Model file for the job. Use its own axes, mm. Face numbers are marked on the shaded views. Coordinates: 2 decimals unless noted, no trailing zeros. Write each loop counter-clockwise with the first axis right and the second up, starting at its lowest first coordinate (ties: lowest second). Pieces come first, ordered by that corner, then holes. Notation, with made-up numbers: (10.5, 80) -> (53.5, 80) arc R16 ccw to (53.5, 94) -> close; hole circle Ø3 at (32.5, -1). An arc over 180 degrees is marked (long way). Answer as a JSON object with one key per item and string values. Group by question number.
from build123d import *

# Parameters (mm, degrees)
SKETCH1_W           = 59.999999888
SKETCH1_H           = 29.999999944
SKETCH1_R           = 6.35889
SKETCH1_R_2         = 2.499999953
BOSS_EXTRUDE1_DEPTH = 6.35
SKETCH2_R           = 9.53389
SKETCH2_R_2         = 6.35889
BOSS_EXTRUDE2_DEPTH = 25.4
FILLET1_R           = 1.27


with BuildPart() as part:
    # Sketch1 → Boss-Extrude1 (new body)
    with BuildSketch(Plane(origin=(0, 0, 0), x_dir=(1, 0, 0), z_dir=(0, 1, 0))):
        Rectangle(SKETCH1_W, SKETCH1_H)
        with Locations(Location((0, 0, 0), (0, 0, 270))):
            Circle(SKETCH1_R, mode=Mode.SUBTRACT)
        with Locations(Location((-25.554999944, 10.554999972, 0), (0, 0, 270))):
            Circle(SKETCH1_R_2, mode=Mode.SUBTRACT)
        with Locations(Location((25.554999944, 10.554999972, 0), (0, 0, 270))):
            Circle(SKETCH1_R_2, mode=Mode.SUBTRACT)
        with Locations(Location((25.554999944, -10.554999972, 0), (0, 0, 270))):
            Circle(SKETCH1_R_2, mode=Mode.SUBTRACT)
        with Locations(Location((-25.554999944, -10.554999972, 0), (0, 0, 270))):
            Circle(SKETCH1_R_2, mode=Mode.SUBTRACT)
    extrude(amount=BOSS_EXTRUDE1_DEPTH)

    # Sketch2 → Boss-Extrude2 (add)
    with BuildSketch(Plane(origin=(0, 6.35, 0), x_dir=(1, 0, 0), z_dir=(0, 1, 0))):
        with Locations(Location((0, 0, 0), (0, 0, 270))):
            Circle(SKETCH2_R)
        with Locations(Location((0, 0, 0), (0, 0, 270))):
            Circle(SKETCH2_R_2, mode=Mode.SUBTRACT)
    extrude(amount=BOSS_EXTRUDE2_DEPTH)

    # Fillet1
    fillet1_edges = [part.edges().sort_by_distance(p)[0] for p in [
        (-29.999999944, 3.175, 14.999999972),
        (-29.999999944, 3.175, -14.999999972),
        (29.999999944, 3.175, -14.999999972),
        (29.999999944, 3.175, 14.999999972),
        (0, 6.35, -9.53389),
        (0, 31.75, -9.53389),
    ]]
    fillet(fillet1_edges, radius=FILLET1_R)

    # Chamfer5: read off the stored shape, not the designer's step
    # Chamfer5 outline → Chamfer5 (revolve, cut)
    with BuildSketch(Plane.XY):
        Polygon((6.35889, 31.75), (6.35889, 31.4325), (6.67639, 31.75), align=None)
    revolve(axis=Axis((0, 0, 0), (0, 1, 0)), mode=Mode.SUBTRACT)


solid = part.part
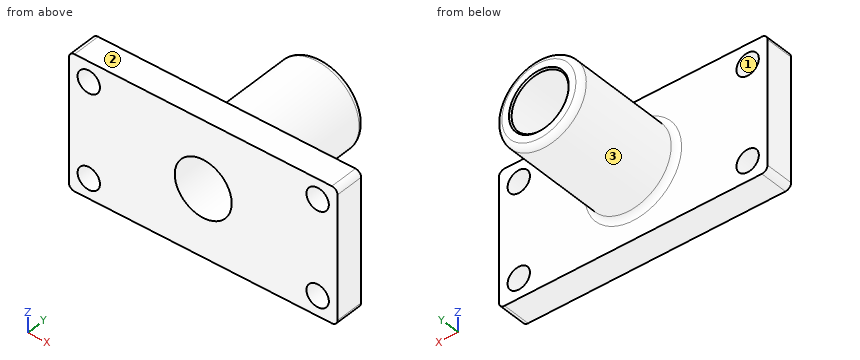
(1) Cut at A-A on x = 0. List the corners of the cut face in (y, z), plus the area to 3 significant figures.
(2) Pin check, flat tips, straight feed: pin 1 (8 mm diameter, centred on y = 10.5, z = 7.5, fed in from -X); pin 2 (4 mm diameter, centred on x = -3.5, y = 21.5, fed in from -Z); pin 3 (3 mm diameter, centred on y = 28.5, z = 7, fed in from -X). Stop position of each tip, or through.
(3) Cut at B-B on z = 0. List the corners of the cut face in (x, y).
(4) Cut at C-C on z = 12. List the corners of the cut face in (x, y).
(5) Cut at D-D on y = 22.5. List the corners of the cut face in (x, z).
(6) Pull direction X, two halves, no side cores. Call the marked faces 1, 2 and 3: released by +X, released by -X, zero draft, split by the parting line, or undercut.
(7) Wall check: probe 1 along Z at (x, y) = (27, 5.5); probe 2 along Y at (x, z) = (14.5, 8.5); probe 3 along X at (y, z) = (21.5, -2.5). Give the ranges that are in metal, low to high.
Results found:
{
 "1": {"outline": "(0, -15) -> (6.35, -15) -> (6.35, -10.8) arc R1.27 cw to (7.62, -9.53) -> (30.48, -9.53) arc R1.27 ccw to (31.75, -8.26) -> (31.75, -6.68) -> (31.43, -6.36) -> (0, -6.36) -> close; (0, 6.36) -> (31.43, 6.36) -> (31.75, 6.68) -> (31.75, 8.26) arc R1.27 ccw to (30.48, 9.53) -> (7.62, 9.53) arc R1.27 cw to (6.35, 10.8) -> (6.35, 15) -> (0, 15) -> close", "area": "271 mm²"},
 "2": {"pin 1": "stops at x = -8.87", "pin 2": "stops at z = -9.42", "pin 3": "stops at x = -7.79"},
 "3": {"outline": "(-30, 0) -> (-6.36, 0) -> (-6.36, 31.43) -> (-6.68, 31.75) -> (-8.26, 31.75) arc R1.27 ccw to (-9.53, 30.48) -> (-9.53, 7.62) arc R1.27 cw to (-10.8, 6.35) -> (-30, 6.35) -> close; (6.36, 0) -> (30, 0) -> (30, 6.35) -> (10.8, 6.35) arc R1.27 cw to (9.53, 7.62) -> (9.53, 30.48) arc R1.27 ccw to (8.26, 31.75) -> (6.68, 31.75) -> (6.36, 31.43) -> close"},
 "4": {"outline": "(-30, 0) -> (-27.6, 0) -> (-27.6, 6.35) -> (-30, 6.35) -> close; (-23.51, 0) -> (23.51, 0) -> (23.51, 6.35) -> (-23.51, 6.35) -> close; (27.6, 0) -> (30, 0) -> (30, 6.35) -> (27.6, 6.35) -> close"},
 "5": {"outline": "circle Ø19.07 at (0, 0); hole circle Ø12.72 at (0, 0)"},
 "6": {"face 1": "undercut", "face 2": "zero draft", "face 3": "split by the parting line"},
 "7": {"probe 1": "z = -15 to -12.6, -8.51 to 8.51, 12.6 to 15", "probe 2": "y = 0 to 6.35", "probe 3": "x = -9.2 to -5.85, 5.85 to 9.2"}
}
